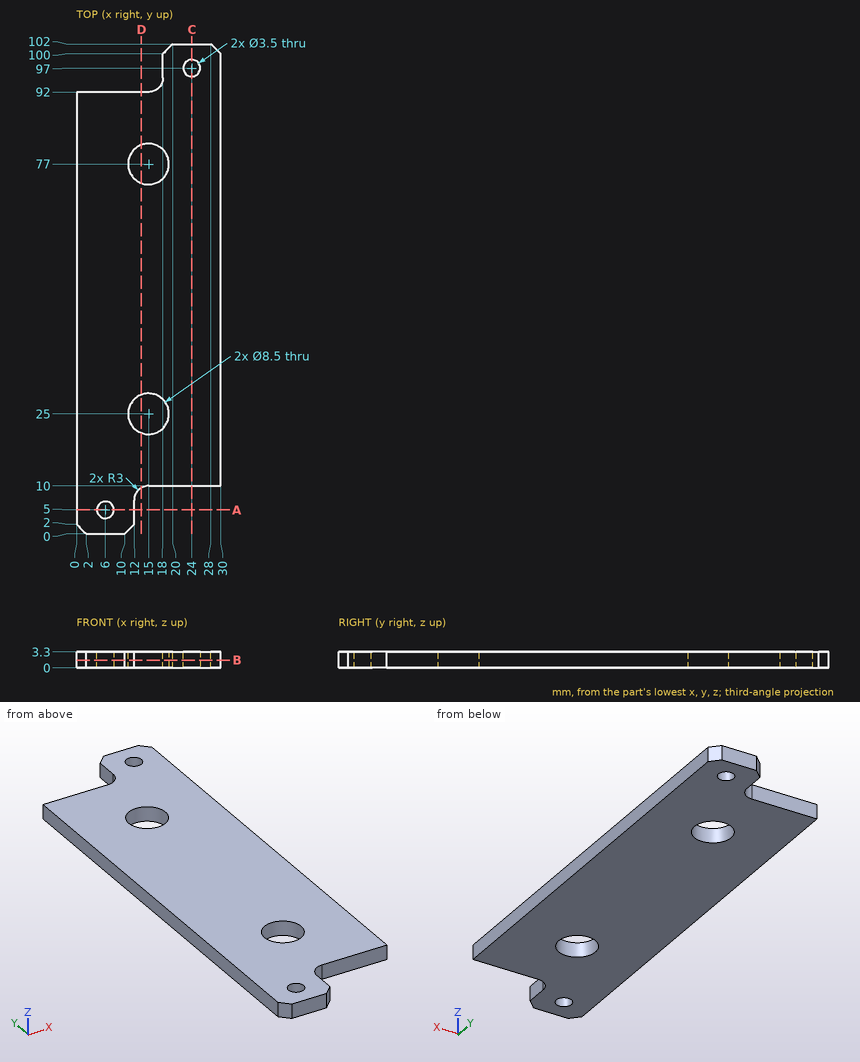
Part print with two shaded views. Sizes in mm from the minimum x, y, z corner. Round coordinates to 2 decimals unless told otherwise and drop trailing zeros. Write each loop counter-clockwise with the first axis right and the second up, starting at its lowest first coordinate (ties: lowest second). Pieces come first, ordered by that corner, then holes. Notation, with made-up numbers: M 86.25,-3 L 106.25,-3 A20 ccw 106.25,11 Z; hole C 22.25,-28 d8. An arc over 180 degrees is marked long. Put each result on its own line as item: value. Start each with the question number.
1) Saw through at D-D, the plane x = 13.5. Write the cut outline in (y, z), and give its area (3 significant figures).
2) Saw through at C-C, the plane x = 24. Write the cut outline in (y, z), and give its area (3 significant figures).
3) Drill centre lines: probe 1 along Y at (x, z) = (15, 2); probe 2 along Y at (x, z) = (6, 0.8); probe 3 along Y at (x, z) = (24, 2.1). Where is each one in solid material? Low to high. Write a range as [from, to].
4) Saw through at A-A, the plane y = 5. Write the cut outline in (x, z).
5) Saw through at B-B, the plane z = 1.6. Write the cut outline in (x, y).
6) Pin check, flat tips, straight feed: pin 1 Ø1.6 at (x, z) = (19.5, 1) entering from -Y; pin 2 Ø1 at (y, z) = (97.5, 1.5) entering from -X; pin 3 Ø1.6 at (x, z) = (7.5, 1.5) entering from +Y. Stop position of each tip, or through.
Resolved:
1. outline: M 9.6,0 L 21.02,0 L 21.02,3.3 L 9.6,3.3 Z; M 28.98,0 L 73.02,0 L 73.02,3.3 L 28.98,3.3 Z; M 80.98,0 L 92,0 L 92,3.3 L 80.98,3.3 Z
1. area: 219 mm²
2. outline: M 10,0 L 95.25,0 L 95.25,3.3 L 10,3.3 Z; M 98.75,0 L 102,0 L 102,3.3 L 98.75,3.3 Z
2. area: 292 mm²
3. probe 1: [10, 20.75], [29.25, 72.75], [81.25, 92]
3. probe 2: [0, 3.25], [6.75, 92]
3. probe 3: [10, 95.25], [98.75, 102]
4. outline: M 0,0 L 4.25,0 L 4.25,3.3 L 0,3.3 Z; M 7.75,0 L 12,0 L 12,3.3 L 7.75,3.3 Z
5. outline: M 0,2 L 2,0 L 10,0 L 12,2 L 12,7 A3 cw 15,10 L 30,10 L 30,100 L 28,102 L 20,102 L 18,100 L 18,95 A3 cw 15,92 L 0,92 Z; hole C 6,5 d3.5; hole C 15,25 d8.5; hole C 15,77 d8.5; hole C 24,97 d3.5
6. pin 1: y = 10
6. pin 2: x = 18
6. pin 3: y = 92
